Geometry: final body of the model. Coordinates: model frame, mm. A direction names the side the tool comes from. Round coordinates to 2 decimals unless told otherwise and drop trailing zeros. Order: outer loops, then holes, each group sorted by start corner. A loop starts at its lowest first (then second) coordinate and runs counter-clockwise, first axis right, second up. Notation, with made-up numbers: M 55.25,85.25 L 108.25,85.25 A21 ccw 108.25,109.25 Z; hole C -31,62.25 d7. An arc over 180 degrees is marked long. Return JSON: item names as keys, results as strings. Group by question number.
Q1. Cut plane D-D on x = 51. Output: boundary loops of the cut face in (y, z), and give its area (3 significant figures).
Q2. Contact query for flat-ended pins moving along their axis: pin 1 (6 mm diameter, centred on x = 45, y = -21, fed in from +Z); pin 2 (5 mm diameter, centred on x = 17, y = -15.5, fed in from -Z); pin 3 (3.5 mm diameter, centred on x = 10, y = -18, fed in from -Z); pin 4 (4 mm diameter, centred on x = 26.5, z = -7, fed in from -Y). Output: stop coordinate, or through.
Q3. Access query for faces 1 (the face through (57.368, -17.156, -4.278)), 2 (the face through (32, -33.679, 2)), 3 (the face through (11, -17, 0)). Directions: +Z, -Z, +X, -X, +Y, -Y. A direction counts if a zero-diameter tool reaches every point of the face in a straight line with its end or side. Return the directions, or none.
Q4. Ray query, probe 1 along Y at (x, z) = (11, 2.75); probe 2 along X at (y, z) = (-9, 1.5); probe 3 along Z at (x, y) = (54, -16). Return the intervals inside material, ascending.
Q5. Cut plane B-B on z = 3.5. Output: boundary loops of the cut face in (x, y).
Q6. Cut plane A-A on x = 11.5. Output: boundary loops of the cut face in (y, z).
```python
from build123d import *

# Parameters (mm, degrees)
F0_W     = 55.4297519848
F0_H     = 34.7989164293
F0_W_2   = 53.9102558978
F0_H_2   = 33.0191702233
F1_DEPTH = 4.572
F2_W     = 54.6025102958
F2_H     = 33.4553048015
F3_DEPTH = 1.27
F5_DEPTH = 34.7989164293
F6_W     = 13.8362795115
F6_H     = 32.7950716601
F7_DEPTH = 8.382


with BuildPart() as f1:
    # F0 (on Top) → F1 (new body)
    with BuildSketch(Plane.XY):
        with Locations((32.8427054919, -17.3994582146)):
            Rectangle(F0_W, F0_H)
        with Locations((32.6169689652, -17.169818253)):
            Rectangle(F0_W_2, F0_H_2, mode=Mode.SUBTRACT)
    extrude(amount=F1_DEPTH)

    # F2 (on Top) → F3 (join)
    with BuildSketch(Plane.XY):
        with Locations((32.2563764639, -16.7276524007)):
            Rectangle(F2_W, F2_H)
    extrude(amount=F3_DEPTH)

    # F4 (on face) → F5 (join, through all)
    with BuildSketch(Plane(origin=(0, 0, 0), x_dir=(-1, 0, 0), z_dir=(0, 1, 0))):
        Polygon((-41.7104549706, 0), (-54.087433964, 0), (-60.5575814843, 0), (-54.087433964, -8.6766919121), (-41.7104549706, -8.6766919121), (-17.0669779181, 0), align=None)
    extrude(amount=-F5_DEPTH)

    # F6 (on face) → F7 (join)
    with BuildSketch(Plane.XY.offset(1.27)):
        with Locations((46.8185357749, -17.0577689714)):
            Rectangle(F6_W, F6_H)
    extrude(amount=-F7_DEPTH)


solid = f1.part
```
Result sheet:
{
 "1": {"outline": "M -34.8,-8.68 L 0,-8.68 L 0,4.57 L -0.66,4.57 L -0.66,1.27 L -33.46,1.27 L -33.46,0 L -33.68,0 L -33.68,4.57 L -34.8,4.57 Z", "area": "352 mm²"},
 "2": {"pin 1": "stops at z = 1.27", "pin 2": "stops at z = -0.86", "pin 3": "stops at z = 0", "pin 4": "passes through"},
 "3": {"face 1": "-Z, +X, +Y, -Y", "face 2": "+Z", "face 3": "-Z, -X, +Y, -Y"},
 "4": {"probe 1": "y = -34.8 to -33.68, -0.66 to 0", "probe 2": "x = 5.13 to 5.66, 59.57 to 60.56", "probe 3": "z = -8.68 to 1.27"},
 "5": {"outline": "M 5.13,-34.8 L 60.56,-34.8 L 60.56,0 L 5.13,0 Z; hole M 5.66,-33.68 L 59.57,-33.68 L 59.57,-0.66 L 5.66,-0.66 Z"},
 "6": {"outline": "M -34.8,0 L -33.68,0 L -33.68,4.57 L -34.8,4.57 Z; M -33.46,0 L 0,0 L 0,4.57 L -0.66,4.57 L -0.66,1.27 L -33.46,1.27 Z"}
}
